```python
from build123d import *

# Parameters (mm, degrees)
SKETCH1_W           = 206.248
SKETCH1_H           = 206.248
C_DIM_DEPTH         = 43.18
SHAFT_START         = 12.7
SKETCH_A_R          = 15.875
SHAFT_DEPTH         = 153.67
SKETCH3_W           = 104.14
SKETCH3_H           = 104.14
BOSS_EXTRUDE3_DEPTH = 99.568
FILLET1_R           = 5.715
FILLET4_R           = 5.715
SKETCH4_R           = 77.597
BOSS_EXTRUDE4_DEPTH = 133.35
BOSS_EXTRUDE4_TAPER = 5
FILLET2_R           = 8.255
SKETCH5_W           = 99.328405226
SKETCH5_H           = 47.124202614
BOSS_EXTRUDE5_DEPTH = 20.32
CHAMFER1_SIZE       = 0.381
FILLET3_R           = 3.175
CUT_EXTRUDE_START   = 12.3698
CUT_EXTRUDE_B_DEPTH = 68.6402


with BuildPart() as part:
    # Sketch1 → C dim (new body)
    with BuildSketch(Plane.XY):
        Rectangle(SKETCH1_W, SKETCH1_H)
    extrude(amount=C_DIM_DEPTH)



with BuildPart() as body_2:
    # Sketch A → Shaft (new body)
    with BuildSketch(Plane(origin=(0, 0, 0), x_dir=(0, 0, -1), z_dir=(1, 0, 0)).offset(SHAFT_START)):
        with Locations((-116.84, 0)):
            Circle(SKETCH_A_R)
    extrude(amount=SHAFT_DEPTH)

    # Chamfer1
    chamfer1_edges = [body_2.edges().sort_by_distance(p)[0] for p in [
        (166.37, 0, 132.715),
    ]]
    chamfer(chamfer1_edges, length=CHAMFER1_SIZE)

    # Sketch6 → Cut-Extrude B (cut, through all)
    with BuildSketch(Plane.XY.offset(116.84).offset(CUT_EXTRUDE_START)):
        with BuildLine():
            Line((166.37, -3.175), (109.093, -3.175))
            ThreePointArc((109.093, -3.175), (105.918, 0), (109.093, 3.175))
            Line((109.093, 3.175), (166.37, 3.175))
            ThreePointArc((166.37, 3.175), (169.545, 0), (166.37, -3.175))
        make_face()
    extrude(amount=CUT_EXTRUDE_B_DEPTH, mode=Mode.SUBTRACT)


with BuildPart() as body_3:
    # Sketch3 → Boss-Extrude3 (new body)
    with BuildSketch(Plane(origin=(0, 0, 0), x_dir=(0, 0, -1), z_dir=(1, 0, 0))):
        with Locations((-116.84, 0)):
            Rectangle(SKETCH3_W, SKETCH3_H)
    extrude(amount=BOSS_EXTRUDE3_DEPTH)


with BuildPart() as body_4:
    # Mirror2: mirrored copy
    add(body_3.part.mirror(Plane(origin=(0, 0, 0), x_dir=(0, 0, 1), z_dir=(1, 0, 0))))

    # Fillet4
    fillet4_edges = [body_4.edges().sort_by_distance(p)[0] for p in [
        (-49.784, 52.07, 64.77),
        (-49.784, 52.07, 168.91),
        (-49.784, -52.07, 168.91),
        (-49.784, -52.07, 64.77),
    ]]
    fillet(fillet4_edges, radius=FILLET4_R)


with BuildPart() as body_3_1:
    add(body_3.part)

    # Fillet1
    fillet1_edges = [body_3_1.edges().sort_by_distance(p)[0] for p in [
        (49.784, 52.07, 64.77),
        (49.784, 52.07, 168.91),
        (49.784, -52.07, 168.91),
        (49.784, -52.07, 64.77),
    ]]
    fillet(fillet1_edges, radius=FILLET1_R)


with BuildPart() as part_1:
    add(part.part)

    add(body_3_1.part)  # Boss-Extrude4 merges body 3

    add(body_4.part)  # Boss-Extrude4 merges body 4
    # Sketch4 → Boss-Extrude4 (add)
    with BuildSketch(Plane.XY.offset(43.18)):
        Circle(SKETCH4_R)
    extrude(amount=BOSS_EXTRUDE4_DEPTH, taper=BOSS_EXTRUDE4_TAPER)

    # Fillet2
    fillet2_edges = [part_1.edges().sort_by_distance(p)[0] for p in [
        (-65.930386719, 0, 176.53),
        (-77.597, 0, 43.18),
        (-103.124, 103.124, 21.59),
        (103.124, 103.124, 21.59),
        (103.124, -103.124, 21.59),
        (-103.124, -103.124, 21.59),
    ]]
    fillet(fillet2_edges, radius=FILLET2_R)

    # Sketch5 → Boss-Extrude5 (add)
    with BuildSketch(Plane.XY.offset(176.53)):
        Rectangle(SKETCH5_W, SKETCH5_H)
    extrude(amount=BOSS_EXTRUDE5_DEPTH)

    # Fillet3
    fillet3_edges = [part_1.edges().sort_by_distance(p)[0] for p in [
        (-49.664202613, 23.562101307, 186.69),
        (-49.664202613, -23.562101307, 186.69),
        (49.664202613, -23.562101307, 186.69),
        (49.664202613, 23.562101307, 186.69),
        (0, 23.562101307, 196.85),
        (-49.664202613, 0, 196.85),
        (0, -23.562101307, 196.85),
        (49.664202613, 0, 196.85),
    ]]
    fillet(fillet3_edges, radius=FILLET3_R)

    # Combine1: union body 2
    add(body_2.part)


solid = part_1.part
```
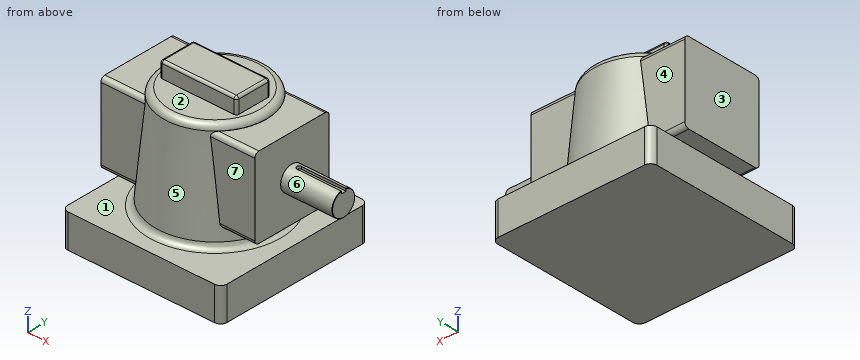
Work out the finished part from the listing and answer in its coordinate system (mm). Face numbers are marked on the shaded views. A direction names the side the tool comes from. Give positions to 0.01 mm unless a question says otherwise; leave off trailing zeros. Loops run counter-clockwise (first coordinate to the right, second up) from the corner with the lowest first, then second, coordinate; pieces in that order, holes last. Notation, with made-up numbers: (39, 85.5) -> (86, 85.5) arc R35 cw to (86, 120.5) -> close; hole circle Ø2 at (83.25, 8). An arc over 180 degrees is marked (long way). Put each result on its own line as item: value. Start each with the question number.
Item 1: The part is cut by section C-C (x = 0). Give the vertices of the cut face in (y, z) (3 decimals).
Item 2: The mould has two halves that part along Z. Classify the marked faces 1, 2 and 3: released by +Z, released by -Z, zero draft, split by the parting line, or undercut.
Item 3: The part is cut by section D-D (z = 28.5). Give the vertices of the cut face in (x, y) (3 decimals).
Item 4: Which of the six approach directions +Z, -Z, +X, -X, +Y, -Y give full straight-line access (tool end or side, diameter ignored) to the marked faces 4, 5, 6 and 7?
Item 5: Find the intervals of material crossed by L1, parallel to Z at x = 97, y = 45.5; L2, parallel to Z at x = 34, y = -46; L3, parallel to Z at x = 10.5, y = 93.5, in increasing order. Write a range as [from, to].
Item 6: Each of these flat-tipped pins is pushed along its axis until it touches: P1, Ø3, axis at x = 8.5, z = 171, coming from the -Y side; P2, Ø3, axis at y = -74.5, z = 41, coming from the +X side; P3, Ø13.5, axis at y = 6, z = 189, coming from the -X side. Where does it stop, or does it pass through?
Item 7: The part is cut by section A-A (x = 89). Give the vertices of the cut face in (y, z) (3 decimals).
Item 8: The part is cut by section B-B (z = 183.5). Give the vertices of the cut face in (x, y) (3 decimals).
Answers below:
1. outline: (-103.124, 0) -> (103.124, 0) -> (103.124, 43.18) -> (85.161, 43.18) arc R8.255 cw to (76.938, 50.716) -> (66.59, 168.994) arc R8.255 ccw to (58.366, 176.53) -> (23.562, 176.53) -> (23.562, 193.675) arc R3.175 ccw to (20.387, 196.85) -> (-20.387, 196.85) arc R3.175 ccw to (-23.562, 193.675) -> (-23.562, 176.53) -> (-58.366, 176.53) arc R8.255 ccw to (-66.59, 168.994) -> (-76.938, 50.716) arc R8.255 cw to (-85.161, 43.18) -> (-103.124, 43.18) -> close
2. face 1: undercut
2. face 2: released by +Z
2. face 3: zero draft
3. outline: (-103.124, -94.869) arc R8.255 ccw to (-94.869, -103.124) -> (94.869, -103.124) arc R8.255 ccw to (103.124, -94.869) -> (103.124, 94.869) arc R8.255 ccw to (94.869, 103.124) -> (-94.869, 103.124) arc R8.255 ccw to (-103.124, 94.869) -> close
4. face 4: +Z, -X, +Y
4. face 5: none
4. face 6: +X
4. face 7: +Z, +X, -Y
5. L1: [0, 43.18], [64.77, 168.91]
5. L2: [0, 176.53]
5. L3: [0, 43.18]
6. P1: y = -66.04
6. P2: x = 103.12
6. P3: x = -49.66
7. outline: (-103.124, 0) -> (103.124, 0) -> (103.124, 43.18) -> (-103.124, 43.18) -> close; (-52.07, 70.485) arc R5.715 ccw to (-46.355, 64.77) -> (46.355, 64.77) arc R5.715 ccw to (52.07, 70.485) -> (52.07, 163.195) arc R5.715 ccw to (46.355, 168.91) -> (-46.355, 168.91) arc R5.715 ccw to (-52.07, 163.195) -> close
8. outline: (-49.664, -20.387) arc R3.175 ccw to (-46.489, -23.562) -> (46.489, -23.562) arc R3.175 ccw to (49.664, -20.387) -> (49.664, 20.387) arc R3.175 ccw to (46.489, 23.562) -> (-46.489, 23.562) arc R3.175 ccw to (-49.664, 20.387) -> close
